The drawing under review shows one solid part. Ordinate dimensions are in mm from its lowest x, y, z. Coordinates: 2 decimals unless noted, no trailing zeros. Write each loop counter-clockwise with the first axis right and the second up, starting at its lowest first coordinate (ties: lowest second). Pieces come first, ordered by that corner, then holes.
Q1. Take a section at C-C (x = 58.5). Give the boundary of the cut face in (y, z).
Q2. For probe 1 along X at (y, z) = (33.5, 6); probe 2 along Y at (x, z) = (79.5, 1.5), list the stretches that pass through material, from the lowest coordinate up.
Q3. Take a section at A-A (y = 27.5). Give the boundary of the cut face in (x, z), and give its area (3 significant figures).
Q4. Take a section at B-B (z = 6). Give the boundary of the cut face in (x, y).
Q5. Insertion check: pin 1 (2 mm diameter, centred on x = 68.5, z = 6, fed in from -Y). The pin has a flat end and moves straight along its axis. Give the tip position at first contact, or say it passes through.
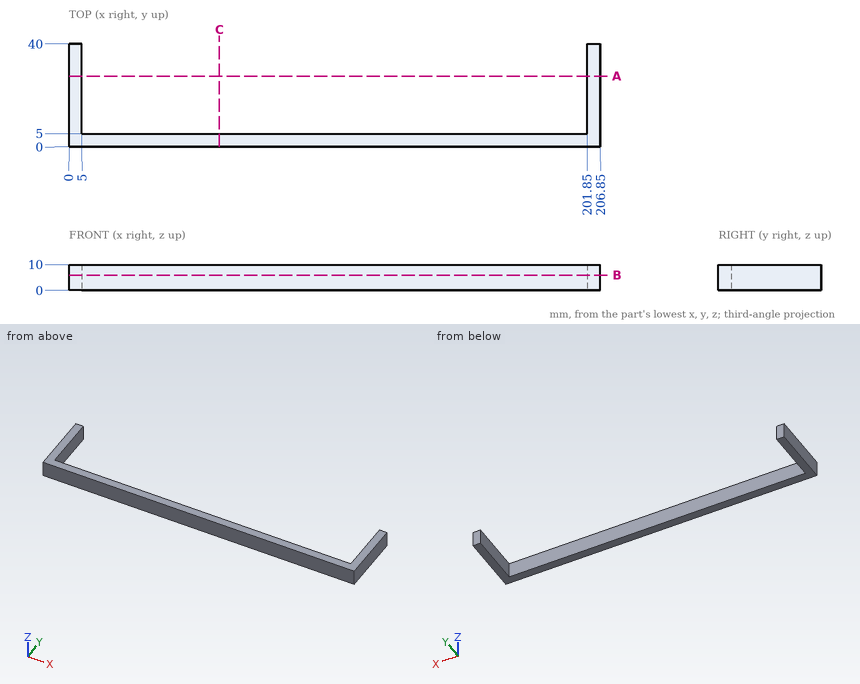
Response:
1. outline: (0, 0) - (5, 0) - (5, 10) - (0, 10) - close
2. probe 1: x = 0 to 5, 201.85 to 206.85
2. probe 2: y = 0 to 5
3. outline: (0, 0) - (5, 0) - (5, 10) - (0, 10) - close; (201.85, 0) - (206.85, 0) - (206.85, 10) - (201.85, 10) - close
3. area: 100 mm2
4. outline: (0, 0) - (206.85, 0) - (206.85, 40) - (201.85, 40) - (201.85, 5) - (5, 5) - (5, 40) - (0, 40) - close
5. pin 1: stops at y = 0
